Autodesk Inventor part; units mm, degrees
ref_plane "YZ Plane" through (0, 0, 0) normal (1, 0, 0) x (0, 1, 0)
ref_plane "XZ Plane" through (0, 0, 0) normal (0, 1, 0) x (-1, 0, 0)
ref_plane "XY Plane" through (0, 0, 0) normal (0, 0, 1) x (1, 0, 0)
sketch "Sketch1" plane through (0, 0, 0) normal (0, 1, 0) x (-1, 0, 0)
  circle A0 centre (0, 0) radius 6
  dimension "d0" = 12
extrude "Extrusion1" add sketch "Sketch1" along normal blind 6 draft 45
extrude "Extrusion2" add sketch "Sketch1" against normal blind 24
chamfer "Chamfer1" distance 2 angle 45 1 edges at (6, -24, 0)
thread "Thread1"
sketch "Sketch2" plane through (0, 6, 0) normal (0, 1, 0) x (1, 0, 0)
  line L0 (1, -12) -> (1, 12)
  line L1 (1, 12) -> (-1, 12)
  line L2 (-1, 12) -> (-1, -12)
  line L3 (-1, -12) -> (1, -12)
  line L4 (1, -12) -> (-1, 12) construction
  line L5 (1, 12) -> (-1, -12) construction
  point P0 (0, 0)
  dimension "d10" = 2
extrude "Extrusion3" cut sketch "Sketch2" against normal blind 3
properties part number "csk.screw" material "Steel, High Strength, Low Alloy"
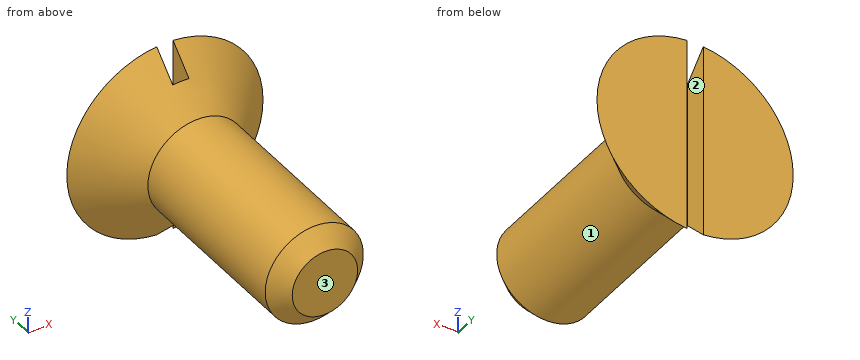
The model under review builds one solid part; all positions refer to its coordinate system, in mm. Face numbers are marked on the shaded views. Round coordinates to 2 decimals unless told otherwise and drop trailing zeros. Order: outer loops, then holes, each group sorted by start corner. A loop starts at its lowest first (then second) coordinate and runs counter-clockwise, first axis right, second up. Notation, with made-up numbers: (32.5, 11) -> (76.5, 11) arc R25 cw to (76.5, 23) -> close; hole circle Ø10 at (80, 25). An arc over 180 degrees is marked (long way). Use a Markdown table: item, result.
Q1. We need section B-B on z = 0. Write out the cut boundary in (x, y).
Values:
| item | result |
|---|---|
| outline | (-12, 6) -> (-6, 0) -> (-6, -22) -> (-4, -24) -> (4, -24) -> (6, -22) -> (6, 0) -> (12, 6) -> (1, 6) -> (1, 3) -> (-1, 3) -> (-1, 6) -> close |
Q2. Clearance check with flat-ended pins moving along their axes: P1, Ø2, axis at x = 4.5, y = -12, coming from the -Z side; P2, Ø0.9, axis at y = 4.5, z = -0.5, coming from the -X side; P3, Ø4, axis at x = 2.5, y = -6, coming from the +Z side. State where each tip first meets the part, or that it passes through.
Values:
| item | result |
|---|---|
| P1 | stops at z = -4.87 |
| P2 | stops at x = -10.94 |
| P3 | stops at z = 5.98 |
Q3. We need section A-A on x = 0. Write out the cut boundary in (y, z).
Values:
| item | result |
|---|---|
| outline | (-24, -4) -> (-22, -6) -> (0, -6) -> (3, -9) -> (3, 9) -> (0, 6) -> (-22, 6) -> (-24, 4) -> close |
Q4. We need section C-C on y = -11. Write out the cut boundary in (x, z).
Values:
| item | result |
|---|---|
| outline | circle Ø12 at (0, 0) |
Q5. For line 1 (Z direction, x = 5.5, y = -4); line 2 (X direction, y = -17, z = -5.25); line 3 (X direction, y = -11, z = 2.5), list the stretches that pass through material, from the lowest coordinate up.
Values:
| item | result |
|---|---|
| line 1 | z = -2.4 to 2.4 |
| line 2 | x = -2.9 to 2.9 |
| line 3 | x = -5.45 to 5.45 |
Q6. Mouldability with a two-part tool opening along X and no side actions: class the marked faces 1, 2 and 3 as +X half, -X half, draft (parallel to the pull), parting line (faces both ways), or undercut.
Values:
| item | result |
|---|---|
| face 1 | parting line |
| face 2 | undercut |
| face 3 | draft |
